CAD build for the part. Positions are in the model's coordinates, mm. A direction names the side the tool comes from. Give positions to 0.01 mm unless a question says otherwise; leave off trailing zeros. Loops run counter-clockwise (first coordinate to the right, second up) from the corner with the lowest first, then second, coordinate; pieces in that order, holes last. Notation, with made-up numbers: (74, 66.25) -> (119, 66.25) arc R26 cw to (119, 101.25) -> close; hole circle Ø4 at (40.25, 77.5). An arc over 180 degrees is marked (long way). Use one line per item in the form item = value.
Solid Edge part; units mm, degrees
sketch "Sketch1" plane through (0, 0, 0) normal (0, -1, 0) x (1, 0, 0)
  line L0 (-69.2402, 30.6087) -> (-35.6398, 30.6102)
  arc A0 (-35.6398, 30.6102) -> (-35.6027, 35.0092) centre (-35.6399, 32.8098) ccw
  line L1 (-35.6027, 35.0092) -> (-69.1679, 35.0077)
  arc A1 (-69.2402, 30.6087) -> (-69.1679, 35.0077) centre (-69.2403, 32.8088) cw
  line L2 (-69.2403, 55.0593) -> (-35.6399, 55.0593)
  arc A2 (-36.3967, 59.4593) -> (-35.6399, 55.0593) centre (-36.3967, 57.1942) cw
  line L3 (-36.3967, 59.4593) -> (-69.2403, 59.4593)
  arc A3 (-69.2403, 55.0593) -> (-69.2403, 59.4593) centre (-69.2403, 57.2593) cw
  line L4 (-27.4403, 49.1944) -> (-27.4403, 25.609)
  line L5 (-68.3891, 25.609) -> (-27.4403, 25.609)
  line L6 (-74.4403, 25.609) -> (-68.3891, 25.609)
  line L7 (-74.4403, 61.6844) -> (-74.4403, 25.609)
  line L8 (-68.3891, 61.6844) -> (-74.4403, 61.6844)
  line L9 (-68.3891, 61.6844) -> (-27.4403, 61.6844)
  line L10 (-27.4403, 49.1944) -> (-27.4403, 61.6844)
extrude "Protrusion1" add sketch "Sketch1" against normal blind 13
1. Cut at C-C, the plane z = 34.5. Write the cut outline in (x, y).
Result sheet:
outline = (-74.44, 0) -> (-70.65, 0) -> (-70.65, 13) -> (-74.44, 13) -> close; (-34.23, 0) -> (-27.44, 0) -> (-27.44, 13) -> (-34.23, 13) -> close
2. Mould opens along X. For faces 3 (the flat face through (-51, 13, 43)), 4 (the flat face through (-74.44, 6, 44)), 5 (the cylindrical face through (-33.44, 6.41, 32.74)) say: pulls with the +X half, pulls with the -X half, needs draft (parallel to the pull), parting line crosses it, or undercut.
Result sheet:
face_3 = needs draft
face_4 = pulls with the -X half
face_5 = undercut
3. Drill centre lines: line 1 (Z direction, x = -37, y = 2); line 2 (Z direction, x = -34.5, y = 12.25); line 3 (X direction, y = 8.5, z = 56). Where is each one in solid material? Low to high.
Result sheet:
line_1 = 25.61 to 30.61, 35.01 to 55.06, 59.46 to 61.68
line_2 = 25.61 to 30.93, 34.69 to 55.96, 58.43 to 61.68
line_3 = -74.44 to -71.04, -34.47 to -27.44
4. Drop a flat-ended pin along its axis: P1, Ø1.5, axis at x = -58, z = 44.5, coming from the -Y side. Give the stop position or say it passes through.
Result sheet:
P1 = 0
5. Cut at B-B, the plane x = -57.5. Write the cut outline in (y, z).
Result sheet:
outline = (0, 25.61) -> (13, 25.61) -> (13, 30.61) -> (0, 30.61) -> close; (0, 35.01) -> (13, 35.01) -> (13, 55.06) -> (0, 55.06) -> close; (0, 59.46) -> (13, 59.46) -> (13, 61.68) -> (0, 61.68) -> close
6. Cut at A-A, the plane y = 10.75. Write the cut outline in (x, z) (3 decimals).
Result sheet:
outline = (-74.44, 25.609) -> (-27.44, 25.609) -> (-27.44, 61.684) -> (-74.44, 61.684) -> close; hole (-69.24, 30.609) -> (-35.64, 30.61) arc R2.2 ccw to (-35.603, 35.009) -> (-69.168, 35.008) arc R2.2 ccw (long way) to start; hole (-69.24, 55.059) -> (-35.64, 55.059) arc R2.265 ccw to (-36.397, 59.459) -> (-69.24, 59.459) arc R2.2 ccw to start
7. Tool access for faces 1 (the cylindrical face through (-34.157, 6.409, 57.534)), 2 (the flat face through (-27.44, 6, 43)): list every direction of +Z, -Z, +X, -X, +Y, -Y with a clear straight run to the whole face (end or side of a thin tool).
Result sheet:
face_1 = +Y, -Y
face_2 = +Z, -Z, +X, +Y, -Y
